The drawing under review shows one solid part. Ordinate dimensions are in mm from its lowest x, y, z. Round coordinates to 2 decimals unless told otherwise and drop trailing zeros. Order: outer loops, then holes, each group sorted by start corner. A loop starts at its lowest first (then second) coordinate and runs counter-clockwise, first axis right, second up. Notation, with made-up numbers: M 60.25,56.5 L 94.25,56.5 A15 ccw 94.25,75.5 Z; hole C 18.5,60 d8. An arc over 180 degrees is marked long. Answer as a JSON object with one key per item and string values. Group by question number.
1) Consider section D-D, the plane x = 13.25. Write out the cut boundary in (y, z) (1 decimal).
2) Insertion check: pin 1 Ø8 at (x, y) = (12, 13.5) entering from -Z; pin 2 Ø3 at (x, y) = (2.5, 3.5) entering from +Z (1 decimal); pin 3 Ø2.5 at (x, y) = (9.017, 9.017) entering from +Z. Each pin has a flat end and moves straight along its axis. Give the tip position at first contact, or say it passes through.
3) Consider section A-A, the plane x = 10. Write out the cut boundary in (y, z) (1 decimal).
4) Consider section C-C, the plane y = 7.5. Write out the cut boundary in (x, z) (1 decimal).
5) The part is to be moulded in two halves that separate along Y. For the marked faces 1, 2 and 3, say which applies: +Y half, -Y half, draft (parallel to the pull), parting line (faces both ways), or undercut.
6) Consider section B-B, the plane z = 1.45. Write out the cut boundary in (x, y) (1 decimal).
7) To check wall thickness, follow line 1 (X direction, y = 9, z = 2.4) (1 decimal); line 2 (Z direction, x = 5.75, y = 14.75) (1 decimal); line 3 (X direction, y = 8.25, z = 1.45) (1 decimal). State the ranges of each line that lie inside material, in increasing order.
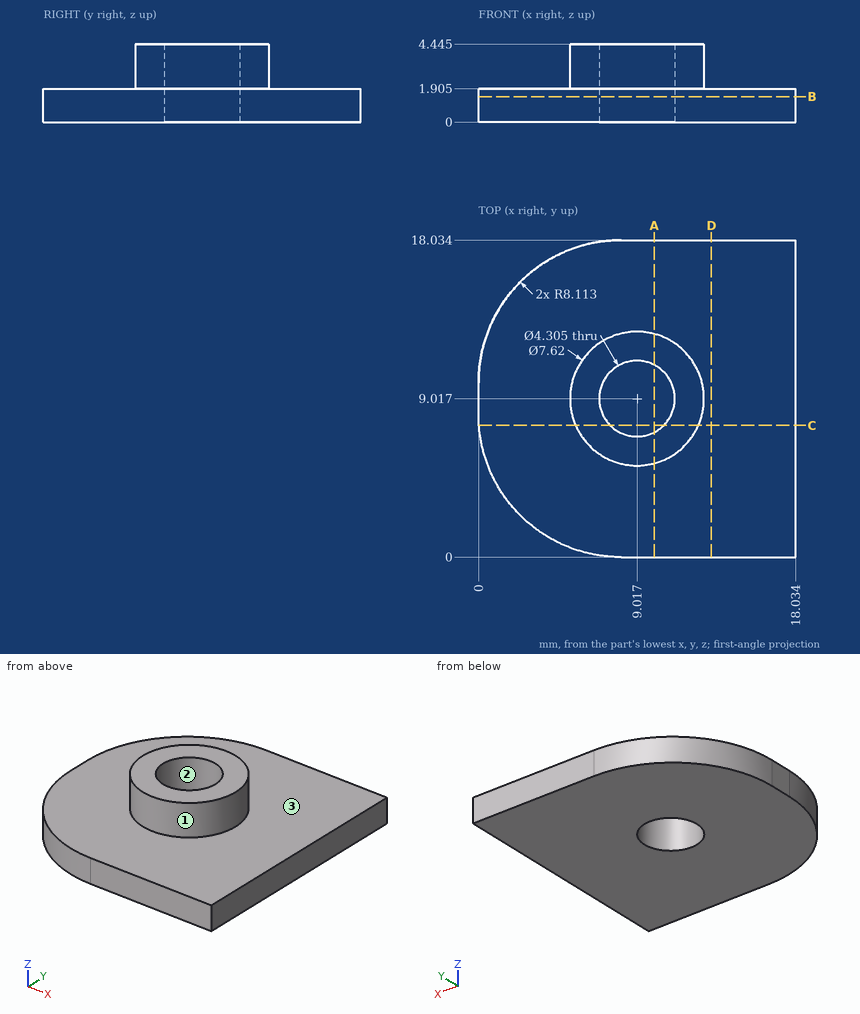
Results list:
{
 "1": {"outline": "M 0,0 L 18,0 L 18,1.9 L 0,1.9 Z"},
 "2": {"pin 1": "z = 0", "pin 2": "z = 1.9", "pin 3": "through"},
 "3": {"outline": "M 0,0 L 7.1,0 L 7.1,4.4 L 5.3,4.4 L 5.3,1.9 L 0,1.9 Z; M 10.9,0 L 18,0 L 18,1.9 L 12.7,1.9 L 12.7,4.4 L 10.9,4.4 Z"},
 "4": {"outline": "M 0,0 L 7.5,0 L 7.5,4.4 L 5.5,4.4 L 5.5,1.9 L 0,1.9 Z; M 10.5,0 L 18,0 L 18,1.9 L 12.5,1.9 L 12.5,4.4 L 10.5,4.4 Z"},
 "5": {"face 1": "parting line", "face 2": "undercut", "face 3": "draft"},
 "6": {"outline": "M 0,8.1 A8.1 ccw 8.1,0 L 18,0 L 18,18 L 8.1,18 A8.1 ccw 0,9.9 Z; hole C 9,9 d4.3"},
 "7": {"line 1": "5.2 to 6.9, 11.2 to 12.8", "line 2": "0 to 1.9", "line 3": "0 to 7, 11 to 18"}
}
